```python
from build123d import *

# Parameters (mm, degrees)
Y_KSEKLIK_EKSTR_ZYON1_DEPTH = 14
IZIM2_R                     = 2
KES_EKSTR_ZYON1_DEPTH       = 14
IZIM3_R                     = 2
KES_EKSTR_ZYON2_DEPTH       = 50


with BuildPart() as part:
    # Çizim1 → Yükseklik-Ekstrüzyon1 (new body)
    with BuildSketch(Plane.XY):
        with BuildLine():
            Line((-58.370675481, 0), (-16.370675481, 0))
            Line((-16.370675481, 0), (-16.370675481, 5))
            ThreePointArc((-16.370675481, 5), (-16.663568699, 5.707106781), (-17.370675481, 6))
            Line((-17.370675481, 6), (-27.370675481, 6))
            ThreePointArc((-27.370675481, 6), (-28.077782262, 6.292893219), (-28.370675481, 7))
            Line((-28.370675481, 7), (-28.370675481, 31.8))
            ThreePointArc((-28.370675481, 31.8), (-28.663568699, 32.507106781), (-29.370675481, 32.8))
            Line((-29.370675481, 32.8), (-35.968113831, 32.8))
            Line((-35.968113831, 32.8), (-35.968113831, 24.746040686))
            ThreePointArc((-35.968113831, 24.746040686), (-37.370675481, 17), (-38.77323713, 24.746040686))
            Line((-38.77323713, 24.746040686), (-38.77323713, 32.8))
            Line((-38.77323713, 32.8), (-45.370675481, 32.8))
            ThreePointArc((-45.370675481, 32.8), (-46.077782262, 32.507106781), (-46.370675481, 31.8))
            Line((-46.370675481, 31.8), (-46.370675481, 7))
            ThreePointArc((-46.370675481, 7), (-46.663568699, 6.292893219), (-47.370675481, 6))
            Line((-47.370675481, 6), (-57.370675481, 6))
            ThreePointArc((-57.370675481, 6), (-58.077782262, 5.707106781), (-58.370675481, 5))
            Line((-58.370675481, 5), (-58.370675481, 0))
        make_face()
    extrude(amount=Y_KSEKLIK_EKSTR_ZYON1_DEPTH)

    # Çizim2 → Kes-Ekstrüzyon1 (cut)
    with BuildSketch(Plane(origin=(0, 6, 0), x_dir=(1, 0, 0), z_dir=(0, 1, 0))):
        with Locations((-22.370675481, -7)):
            Circle(IZIM2_R)
        with Locations((-52.370675481, -7)):
            Circle(IZIM2_R)
    extrude(amount=-KES_EKSTR_ZYON1_DEPTH, mode=Mode.SUBTRACT)

    # Çizim3 → Kes-Ekstrüzyon2 (cut)
    with BuildSketch(Plane(origin=(-28.370675481, 0, 0), x_dir=(0, 0, -1), z_dir=(1, 0, 0))):
        with Locations((-7.037491544, 28)):
            Circle(IZIM3_R)
    extrude(amount=-KES_EKSTR_ZYON2_DEPTH, mode=Mode.SUBTRACT)


solid = part.part
```
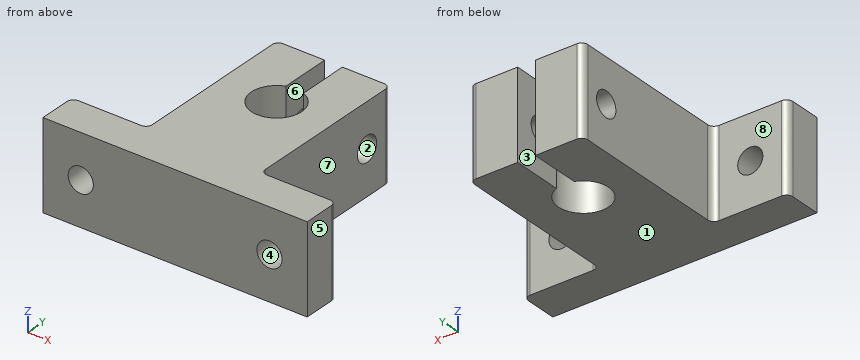
Geometry check sheet. Reference: the model listing, model coordinates, mm. Face numbers are marked on the shaded views. A direction names the side the tool comes from. Coordinates: 2 decimals unless noted, no trailing zeros. Order: outer loops, then holes, each group sorted by start corner. A loop starts at its lowest first (then second) coordinate and runs counter-clockwise, first axis right, second up. Notation, with made-up numbers: M 59.5,-26.75 L 71.5,-26.75 A7 cw 71.5,-16.75 Z; hole C 69.25,45 d9. An arc over 180 degrees is marked long. Answer as a JSON object with one key per item and string values.
Q1. Depth check by flat-ended pin: pin 1 Ø2.5 at (y, z) = (28, 7.04) entering from +X; pin 2 Ø6.5 at (y, z) = (28.5, 9.5) entering from -X; pin 3 Ø3 at (y, z) = (25.5, 7.5) entering from +X. Enter the tip coordinate at first touch or a pass-through.
Results are:
{"pin 1": "passes through", "pin 2": "stops at x = -46.37", "pin 3": "stops at x = -28.37"}
Q2. Tool access check on the marked faces 5, 6, 7 and 8. Record the directions out of +Z, -Z, +X, -X, +Y, -Y that give a thin tool (end or side, any length) a straight path to the whole face; none if there is none.
Results are:
{"face 5": "+Z, -Z, +X, +Y, -Y", "face 6": "+Z, -Z, +Y", "face 7": "+Z, -Z, +X, +Y", "face 8": "+Z, -Z, -X, +Y"}
Q3. Release check for a two-part mould opening along Z. For the marked faces 1, 2, 3 and 4 record: released by +Z, released by -Z, zero draft, split by the parting line, or undercut.
Results are:
{"face 1": "released by -Z", "face 2": "undercut", "face 3": "zero draft", "face 4": "undercut"}
Q4. Cross-section at D-D on x = -32. Record the cut outline in (y, z).
Results are:
{"outline": "M 0,0 L 32.8,0 L 32.8,14 L 0,14 Z; hole C 28,7.04 d4"}
Q5. Cross-section at B-B on z = 8.5. Give the number of separate pieces and of enclosed holes in the cut face, and give its area (3 significant figures).
Results are:
{"separate pieces": "5", "enclosed holes": "0", "area": "588 mm²"}
Q6. Cross-section at A-A on y = 21. Record the cut outline in (x, z).
Results are:
{"outline": "M -46.37,0 L -41.37,0 L -41.37,14 L -46.37,14 Z; M -33.37,0 L -28.37,0 L -28.37,14 L -33.37,14 Z"}
Q7. Scan lines: line 1 (X direction, y = 21, z = 3.75); line 2 (Y direction, x = -25, z = 2.75); line 3 (X direction, y = 3, z = 8). Record each from-to range of solid material in increasing order.
Results are:
{"line 1": "x = -46.37 to -41.37, -33.37 to -28.37", "line 2": "y = 0 to 6", "line 3": "x = -58.37 to -54.1, -50.64 to -24.1, -20.64 to -16.37"}
Q8. Cross-section at C-C on y = 28. Record the cut outline in (x, z).
Results are:
{"outline": "M -46.37,0 L -38.77,0 L -38.77,5.04 L -46.37,5.04 Z; M -46.37,9.04 L -38.77,9.04 L -38.77,14 L -46.37,14 Z; M -35.97,0 L -28.37,0 L -28.37,5.04 L -35.97,5.04 Z; M -35.97,9.04 L -28.37,9.04 L -28.37,14 L -35.97,14 Z"}
